Input: part model. Units: mm. Frame: model coordinates. A direction names the side the tool comes from. Coordinates: 2 decimals unless noted, no trailing zeros. Order: outer loops, then holes, each group sorted by start corner. A loop starts at its lowest first (then second) coordinate and runs counter-clockwise, first axis right, second up. Notation, with made-up numbers: (-34.75, -4) - (-23.75, -4) arc R28 ccw to (-23.75, 32) - close; hole circle Ø4 at (62, -9.75). An arc over 180 degrees is marked (long way). Use a Markdown table: item, result. Add a question column.
from build123d import *

# Parameters (mm, degrees)
SKETCH_W        = 327
SKETCH_H        = 420
PAD_DEPTH       = 3
SKETCH001_R     = 2
POCKET_DEPTH    = 3.001
POCKET001_DEPTH = 3.001


with BuildPart() as part:
    # Sketch → Pad (new body)
    with BuildSketch(Plane.YZ):
        with Locations((0, -17.5)):
            Rectangle(SKETCH_W, SKETCH_H)
    extrude(amount=PAD_DEPTH)

    # Sketch001 (on Face6 of Pad) → Pocket (cut, through all)
    with BuildSketch(Plane.YZ.offset(3)):
        with Locations((-118.5, 182.5)):
            Circle(SKETCH001_R)
        with Locations((118.5, 182.5)):
            Circle(SKETCH001_R)
        with Locations((-118.5, -182.5)):
            Circle(SKETCH001_R)
        with Locations((118.5, -182.5)):
            Circle(SKETCH001_R)
    extrude(amount=-POCKET_DEPTH, mode=Mode.SUBTRACT)

    # Sketch002 (on Face5 of Pocket) → Pocket001 (cut, through all)
    with BuildSketch(Plane.YZ.offset(3)):
        with BuildLine():
            Line((-110, -227.5), (110, -227.5))
            Line((110, -227.5), (100.928932, -218.428932))
            ThreePointArc((100.928932, -218.428932), (97.684699, -216.261205), (93.857864, -215.5))
            Line((93.857864, -215.5), (-93.857864, -215.5))
            ThreePointArc((-93.857864, -215.5), (-97.684699, -216.261205), (-100.928932, -218.428932))
            Line((-100.928932, -218.428932), (-110, -227.5))
        make_face()
    extrude(amount=-POCKET001_DEPTH, mode=Mode.SUBTRACT)


solid = part.part
1) Material intervals for L1, parallel to Y at x = 0.75, z = -182.5; L2, parallel to Z at x = 1.4, y = 118.5; L3, parallel to Z at x = 0.45, y = -49, sorted ascending.
2) Pull-direction query (Y, two-part tool) for faces 3 (the flat face through (1.5, -105.4, -222.9)), 4 (the flat face through (3, -2, -15)); classes: pulls with the +Y half, pulls with the -Y half, needs draft (parallel to the pull), parting line crosses it, or undercut.
3) Cut plane B-B (y = -29.5). Return the cut outline in (x, z).
4) Cut plane A-A (x = 1.95). Return the cut outline in (y, z).
5) Reachability of faces 1 (the flat face through (0, -2, -15)), 2 (the flat face through (1.5, 105.5, -223)) from +Z, -Z, +X, -X, +Y, -Y: full face, straight path, thin tool, end or side. Return the list, or none.
6) Contact query for a flat-ended pin moving along its axis: P1, Ø0.9, axis at x = 1.5, y = 45.5, coming from the -Z side. Output: stop coordinate, or through.
Computed:
| question | item | result |
|---|---|---|
| 1 | L1 | y = -163.5 to -120.5, -116.5 to 116.5, 120.5 to 163.5 |
| 1 | L2 | z = -227.5 to -184.5, -180.5 to 180.5, 184.5 to 192.5 |
| 1 | L3 | z = -215.5 to 192.5 |
| 2 | face 3 | undercut |
| 2 | face 4 | needs draft |
| 3 | outline | (0, -215.5) - (3, -215.5) - (3, 192.5) - (0, 192.5) - close |
| 4 | outline | (-163.5, -227.5) - (-110, -227.5) - (-100.93, -218.43) arc R10 cw to (-93.86, -215.5) - (93.86, -215.5) arc R10 cw to (100.93, -218.43) - (110, -227.5) - (163.5, -227.5) - (163.5, 192.5) - (-163.5, 192.5) - close; hole circle Ø4 at (-118.5, -182.5); hole circle Ø4 at (-118.5, 182.5); hole circle Ø4 at (118.5, -182.5); hole circle Ø4 at (118.5, 182.5) |
| 5 | face 1 | +Z, -Z, -X, +Y, -Y |
| 5 | face 2 | -Z, +X, -X |
| 6 | P1 | stops at z = -215.5 |
